Verification items for the finished model (mm, model axes). A direction names the side the tool comes from. Give positions to 0.01 mm unless a question says otherwise; leave off trailing zeros. Write each loop counter-clockwise with the first axis right and the second up, starting at its lowest first coordinate (ties: lowest second). Pieces come first, ordered by that corner, then holes. Notation, with made-up numbers: (33, 44) -> (65, 44) arc R14 ccw to (65, 66) -> close; hole circle Ø5 at (32, -28.75). An arc over 180 degrees is marked (long way). Answer as CSV lines item,"result". Start each with the question number.
1) Sectioned sample at C-C on x = 5. Give the number of separate pieces and of enclosed holes in the cut face, and give its area (3 significant figures).
2) Gauge pin test, flat ends, axial feed: pin 1 Ø1 at (y, z) = (10.5, -33.5) entering from -X; pin 2 Ø5.5 at (x, z) = (24.5, -11) entering from +Y; pin 3 Ø4 at (x, y) = (26, 15.5) entering from +Z. Record the tip position at first contact, or that the pin passes through.
3) Sectioned sample at A-A on y = 21. Record the cut outline in (x, z).
4) Sectioned sample at B-B on z = -7. Record the cut outline in (x, y).
5) Material ranges on L1, parallel to X at y = 19, z = -47; L2, parallel to Z at x = 45, y = 27.5; L3, parallel to X at y = 11, z = -48, recorded low to high.
6) Mould release check, pull along X, two halves, no side actions. Record for faces 1 (the cylindrical face through (5, 18, -44)), 2 (the flat face through (0, 7, -33)), 3 (the cylindrical face through (47.03, 17.55, -44.79)), 4 (the flat face through (25, 38, -37)): released by +X, released by -X, zero draft, split by the parting line, or undercut.
7) Sectioned sample at D-D on z = -33. Record the cut outline in (x, y).
8) Tool access check on faces 5 (the flat face through (25, 23, -52)), 6 (the cylindrical face through (1.479, 15.461, -13.642)), 7 (the flat face through (25, 6, 0)). Record the directions out of +Z, -Z, +X, -X, +Y, -Y that give a thin tool (end or side, any length) a straight path to the whole face; none if there is none.
```python
from build123d import *

# Parameters (mm, degrees)
SKETCH1_R                                         = 10
BOSS_EXTRUDE1_DEPTH                               = 50
FILLET1_R                                         = 1
SKETCH2_R                                         = 3
CUT_EXTRUDE1_DEPTH                                = 50
SKETCH3_R                                         = 3
CUT_EXTRUDE2_DEPTH                                = 85.243694126
CSK_FOR_8_FLAT_HEAD_MACHINE_SCREW_100_D           = 4.4958
CSK_FOR_8_FLAT_HEAD_MACHINE_SCREW_100_CSINK_D     = 8.4328
CSK_FOR_8_FLAT_HEAD_MACHINE_SCREW_100_CSINK_ANGLE = 100
CSK_FOR_6_FLAT_HEAD_MACHINE_SCREW_100_D           = 3.7973
CSK_FOR_6_FLAT_HEAD_MACHINE_SCREW_100_CSINK_D     = 7.0866
CSK_FOR_6_FLAT_HEAD_MACHINE_SCREW_100_CSINK_ANGLE = 100
SKETCH14_R                                        = 14.687199229
CUT_EXTRUDE3_DEPTH                                = 3
SKETCH15_R                                        = 14.460805981
CUT_EXTRUDE4_DEPTH                                = 3


with BuildPart() as part:
    # Sketch1 → Boss-Extrude1 (new body)
    with BuildSketch(Plane(origin=(0, 0, 0), x_dir=(0, 0, -1), z_dir=(1, 0, 0))):
        Polygon((53, 0), (54, 1), (54, 11), (52, 13), (52, 35), (40, 35), (34, 41), (20, 41), (14, 35), (2, 35), (2, 13), (0, 11), (0, 1), (1, 0), (18, 0), (19, 1), (35, 1), (36, 0), align=None)
        with Locations((27, 21)):
            Circle(SKETCH1_R, mode=Mode.SUBTRACT)
    extrude(amount=BOSS_EXTRUDE1_DEPTH)

    # Fillet1
    fillet1_edges = [part.edges().sort_by_distance(p)[0] for p in [
        (25, 35, -2),
        (25, 35, -52),
    ]]
    fillet(fillet1_edges, radius=FILLET1_R)

    # Sketch2 → Cut-Extrude1 (cut)
    with BuildSketch(Plane.XZ):
        with Locations(Location((5, -7, 0), (0, 0, 270))):
            Circle(SKETCH2_R)
        with Locations(Location((45, -7, 0), (0, 0, 270))):
            Circle(SKETCH2_R)
    extrude(amount=-CUT_EXTRUDE1_DEPTH, mode=Mode.SUBTRACT)

    # Sketch3 → Cut-Extrude2 (cut, through all)
    with BuildSketch(Plane.XZ):
        with Locations(Location((5, -47, 0), (0, 0, 270))):
            Circle(SKETCH3_R)
        with Locations(Location((45, -47, 0), (0, 0, 270))):
            Circle(SKETCH3_R)
    extrude(amount=-CUT_EXTRUDE2_DEPTH, mode=Mode.SUBTRACT)

    # CSK for #8 Flat Head Machine Screw (100)1 (through all)
    with Locations(Plane(origin=(0, 0, 0), x_dir=(-1, 0, 0), z_dir=(0, -1, 0))):
        with Locations((-45, 7), (-5, 7), (-5, 47), (-45, 47)):
            CounterSinkHole(CSK_FOR_8_FLAT_HEAD_MACHINE_SCREW_100_D / 2, CSK_FOR_8_FLAT_HEAD_MACHINE_SCREW_100_CSINK_D / 2, counter_sink_angle=CSK_FOR_8_FLAT_HEAD_MACHINE_SCREW_100_CSINK_ANGLE)

    # CSK for #6 Flat Head Machine Screw (100)1 (through all)
    with Locations(Plane(origin=(0, 35, 0), x_dir=(1, 0, 0), z_dir=(0, 1, 0))):
        with Locations((5, 47), (45, 47), (45, 7), (5, 7)):
            CounterSinkHole(CSK_FOR_6_FLAT_HEAD_MACHINE_SCREW_100_D / 2, CSK_FOR_6_FLAT_HEAD_MACHINE_SCREW_100_CSINK_D / 2, counter_sink_angle=CSK_FOR_6_FLAT_HEAD_MACHINE_SCREW_100_CSINK_ANGLE)

    # Sketch14 → Cut-Extrude3 (cut)
    with BuildSketch(Plane(origin=(50, 0, 0), x_dir=(0, 0, -1), z_dir=(1, 0, 0))):
        with Locations((27, 21)):
            Circle(SKETCH14_R)
    extrude(amount=-CUT_EXTRUDE3_DEPTH, mode=Mode.SUBTRACT)

    # Sketch15 → Cut-Extrude4 (cut)
    with BuildSketch(Plane.ZY):
        with Locations((-27, 21)):
            Circle(SKETCH15_R)
    extrude(amount=-CUT_EXTRUDE4_DEPTH, mode=Mode.SUBTRACT)


solid = part.part
```
Ans:
1,separate pieces,"3"
1,enclosed holes,"1"
1,area,"1,160 mm²"
2,pin 1,"stops at x = 3"
2,pin 2,"stops at y = 35"
2,pin 3,"stops at z = -2"
3,outline,"(0, -52) -> (50, -52) -> (50, -41.69) -> (47, -41.69) -> (47, -37) -> (3, -37) -> (3, -41.46) -> (0, -41.46) -> close; (0, -12.54) -> (3, -12.54) -> (3, -17) -> (47, -17) -> (47, -12.31) -> (50, -12.31) -> (50, -2) -> (0, -2) -> close; hole circle Ø6 at (5, -47); hole circle Ø6 at (5, -7); hole circle Ø6 at (45, -47); hole circle Ø6 at (45, -7)"
4,outline,"(0, 0) -> (0.78, 0) -> (2, 1.02) -> (2, 34.54) -> (1.46, 35) -> (0, 35) -> close; (8, 1.02) -> (9.22, 0) -> (40.78, 0) -> (42, 1.02) -> (42, 34.54) -> (41.46, 35) -> (8.54, 35) -> (8, 34.54) -> close; (48, 1.02) -> (49.22, 0) -> (50, 0) -> (50, 35) -> (48.54, 35) -> (48, 34.54) -> close"
5,L1,"x = 0 to 2, 8 to 42, 48 to 50"
5,L2,"z = -52 to -50, -44 to -34.6, -19.4 to -10, -4 to -2"
5,L3,"x = 0 to 2.17, 7.83 to 42.17, 47.83 to 50"
6,face 1,"undercut"
6,face 2,"released by -X"
6,face 3,"undercut"
6,face 4,"zero draft"
7,outline,"(0, 1) -> (50, 1) -> (50, 7.59) -> (47, 7.59) -> (47, 13) -> (3, 13) -> (3, 7.84) -> (0, 7.84) -> close; (0, 34.16) -> (3, 34.16) -> (3, 29) -> (47, 29) -> (47, 34.41) -> (50, 34.41) -> (50, 41) -> (0, 41) -> close"
8,face 5,"-Z, +X, -X, +Y"
8,face 6,"-X"
8,face 7,"+Z, +X, -X, +Y, -Y"
